Verification items for the finished model (mm, model axes). Face numbers are marked on the shaded views. Round coordinates to 2 decimals unless told otherwise and drop trailing zeros. Write each loop counter-clockwise with the first axis right and the second up, starting at its lowest first coordinate (ties: lowest second). Pieces come first, ordered by that corner, then holes. Notation, with made-up numbers: M -26,56.25 L -5,56.25 A12 ccw -5,70.25 Z; hole C 29,-8 d1. An arc over 180 degrees is marked long. One line per question, with ' | ' between items.
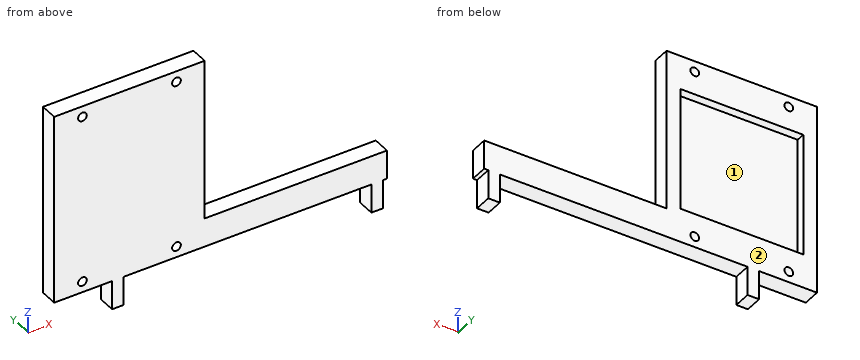
from build123d import *

# Parameters (mm, degrees)
SKETCH1_W           = 52
SKETCH1_H           = 66
BOSS_EXTRUDE1_DEPTH = 6
SKETCH2_W           = 42.5
SKETCH2_H           = 42.5
CUT_EXTRUDE1_DEPTH  = 3
SKETCH3_R           = 1.5
CUT_EXTRUDE2_DEPTH  = 13
SKETCH4_W           = 10
SKETCH4_H           = 6
BOSS_EXTRUDE2_DEPTH = 63
SKETCH5_W           = 4
SKETCH5_H           = 6
BOSS_EXTRUDE3_DEPTH = 10


with BuildPart() as part:
    # Sketch1 → Boss-Extrude1 (new body)
    with BuildSketch(Plane(origin=(0, 0, 0), x_dir=(1, 0, 0), z_dir=(0, 1, 0))):
        with Locations((-26, -33)):
            Rectangle(SKETCH1_W, SKETCH1_H)
    extrude(amount=BOSS_EXTRUDE1_DEPTH)

    # Sketch2 → Cut-Extrude1 (cut)
    with BuildSketch(Plane(origin=(0, 6, 0), x_dir=(1, 0, 0), z_dir=(0, 1, 0))):
        with Locations((-26, -33)):
            Rectangle(SKETCH2_W, SKETCH2_H)
    extrude(amount=-CUT_EXTRUDE1_DEPTH, mode=Mode.SUBTRACT)

    # Sketch3 → Cut-Extrude2 (cut)
    with BuildSketch(Plane(origin=(0, 6, 0), x_dir=(1, 0, 0), z_dir=(0, 1, 0))):
        with Locations(Location((-42.25, -3.75, 0), (0, 0, 270))):
            Circle(SKETCH3_R)
        with Locations(Location((-9.75, -3.75, 0), (0, 0, 90))):
            Circle(SKETCH3_R)
        with Locations(Location((-9.75, -62.25, 0), (0, 0, 270))):
            Circle(SKETCH3_R)
        with Locations(Location((-42.25, -62.25, 0), (0, 0, 90))):
            Circle(SKETCH3_R)
    extrude(amount=-CUT_EXTRUDE2_DEPTH, mode=Mode.SUBTRACT)

    # Sketch4 → Boss-Extrude2 (add)
    with BuildSketch(Plane(origin=(0, 0, 0), x_dir=(0, 0, -1), z_dir=(1, 0, 0))):
        with Locations((-5, 3)):
            Rectangle(SKETCH4_W, SKETCH4_H)
    extrude(amount=BOSS_EXTRUDE2_DEPTH)

    # Sketch5 → Boss-Extrude3 (add)
    with BuildSketch(Plane(origin=(0, 0, 0), x_dir=(-1, 0, 0), z_dir=(0, 0, -1))):
        with Locations((30, 3)):
            Rectangle(SKETCH5_W, SKETCH5_H)
        with Locations((-59.6, 3)):
            Rectangle(SKETCH5_W, SKETCH5_H)
    extrude(amount=BOSS_EXTRUDE3_DEPTH)


solid = part.part
1. Go/stop test with flat-tipped pins: P1, Ø3, axis at y = 3, z = 17.5, coming from the +X side; P2, Ø2.5, axis at x = -42.25, z = 62.25, coming from the -Y side; P3, Ø2, axis at x = 15, y = 2.5, coming from the +Z side; P4, Ø1.8, axis at x = 10.5, y = 2, coming from the -Z side. Record where each tip stops, or that it passes through.
Results:
P1: stops at x = 0 | P2: passes through | P3: stops at z = 10 | P4: stops at z = 0
2. Section check C-C, the plane x = -9.75. Record the cut outline in (y, z), then the cut area to 4 significant figures.
Results:
outline: M 0,0 L 6,0 L 6,2.25 L 0,2.25 Z; M 0,5.25 L 6,5.25 L 6,11.75 L 3,11.75 L 3,54.25 L 6,54.25 L 6,60.75 L 0,60.75 Z; M 0,63.75 L 6,63.75 L 6,66 L 0,66 Z | area: 232.5 mm2
3. Section check A-A, the plane z = 3.75. Record the cut outline in (x, y).
Results:
outline: M -52,0 L -43.75,0 L -43.75,6 L -52,6 Z; M -40.75,0 L -11.25,0 L -11.25,6 L -40.75,6 Z; M -8.25,0 L 63,0 L 63,6 L -8.25,6 Z
4. Section check D-D, the plane z = 42.5. Record the cut outline in (x, y), then the cut area to 4 significant figures.
Results:
outline: M -52,0 L 0,0 L 0,6 L -4.75,6 L -4.75,3 L -47.25,3 L -47.25,6 L -52,6 Z | area: 184.5 mm2
5. Thickness scan on line 1 (X direction, y = 3.6, z = 3.75); line 2 (X direction, y = 3.4, z = 62.25); line 3 (X direction, y = 2, z = 23). Record the ranges inside material, lowest first.
Results:
line 1: x = -52 to -43.75, -40.75 to -11.25, -8.25 to 63 | line 2: x = -52 to -43.75, -40.75 to -11.25, -8.25 to 0 | line 3: x = -52 to 0
6. Mould release check, pull along X, two halves, no side actions. Record for the marked faces 1 and 2: pulls with the +X half, pulls with the -X half, needs draft (parallel to the pull), parting line crosses it, or undercut.
Results:
face 1: undercut | face 2: needs draft
7. Section check B-B, the plane y = 1.6. Record the cut outline in (x, z), then the cut area to 3 significant figures.
Results:
outline: M -52,0 L -32,0 L -32,-10 L -28,-10 L -28,0 L 57.6,0 L 57.6,-10 L 61.6,-10 L 61.6,0 L 63,0 L 63,10 L 0,10 L 0,66 L -52,66 Z; hole C -42.25,3.75 d3; hole C -42.25,62.25 d3; hole C -9.75,3.75 d3; hole C -9.75,62.25 d3 | area: 4,110 mm2
